from build123d import *

# Parameters (mm, degrees)
SKETCH1_W           = 20.32
SKETCH1_H           = 15.24
BOSS_EXTRUDE1_DEPTH = 5.4102
SKETCH2_W           = 10.414
SKETCH2_H           = 2.54
BOSS_EXTRUDE2_DEPTH = 8.382
SKETCH3_R           = 0.5715
CUT_EXTRUDE1_DEPTH  = 5.4102


with BuildPart() as part:
    # Sketch1 → Boss-Extrude1 (new body)
    with BuildSketch(Plane(origin=(0, 0, 0), x_dir=(1, 0, 0), z_dir=(0, 1, 0))):
        with Locations((10.16, 7.62)):
            Rectangle(SKETCH1_W, SKETCH1_H)
    extrude(amount=BOSS_EXTRUDE1_DEPTH)

    # Sketch2 → Boss-Extrude2 (add)
    with BuildSketch(Plane(origin=(0, 5.4102, 0), x_dir=(1, 0, 0), z_dir=(0, 1, 0))):
        with Locations((10.16, 12.7254)):
            Rectangle(SKETCH2_W, SKETCH2_H)
        with Locations((10.16, 2.5146)):
            Rectangle(SKETCH2_W, SKETCH2_H)
    extrude(amount=BOSS_EXTRUDE2_DEPTH)

    # Sketch3 → Cut-Extrude1 (cut)
    with BuildSketch(Plane.XZ):
        with Locations(Location((4.2545, -1.8161, 0), (0, 0, 270))):
            Circle(SKETCH3_R)
        with Locations(Location((16.0655, -1.8161, 0), (0, 0, 270))):
            Circle(SKETCH3_R)
        with Locations(Location((16.0655, -13.4239, 0), (0, 0, 270))):
            Circle(SKETCH3_R)
        with Locations(Location((4.2545, -13.4239, 0), (0, 0, 270))):
            Circle(SKETCH3_R)
    extrude(amount=-CUT_EXTRUDE1_DEPTH, mode=Mode.SUBTRACT)


solid = part.part
Here's how the part is built. I have some questions about the finished solid (model axes, mm). A direction names the side the tool comes from. Round coordinates to 2 decimals unless told otherwise and drop trailing zeros. Write each loop counter-clockwise with the first axis right and the second up, starting at its lowest first coordinate (ties: lowest second). Pieces come first, ordered by that corner, then holes.
1. Will these pins go through, and if not, where does the flat tip stop? pin 1 Ø4 at (x, y) = (9.5, 11.5) entering from -Z; pin 2 Ø0.8 at (y, z) = (9, -12.5) entering from -X; pin 3 Ø2.5 at (x, y) = (10.5, 8.5) entering from +Z.
2. Suppose I cut it at D-D (x = 4). List the corners of the cut face in (y, z) for me, and give its area (3 significant figures).
3. I need wall thicknesses on L1, parallel to Z at x = 5, y = 6.5; L2, parallel to Y at x = 6, z = -8.75. Which ranges of each line are inside material? Lowest first, please.
4. Suppose I cut it at B-B (x = 11.25). List the corners of the cut face in (y, z) for me, and give its area (3 significant figures).
5. For faces 4 (the flat face through (4.953, 10, -13)), 5 (the flat face through (15.367, 10, -13)), 6 (the flat face through (10, 10, -13.995)), 7 (the flat face through (10, 10, -1.245)), 8 (the flat face through (10, 10, -11.455)), which set-ups out of +Z, -Z, +X, -X, +Y, -Y let a thin tool reach every point of the face, with its end or its side?
6. If we mould it in two halves opening along Z, with no side actions, what happens to faces 1 (the flat face through (15.367, 10, -2)), 2 (the flat face through (10, 5.41, -8)), 3 (the flat face through (10, 3, 0))? For each: released by +Z, released by -Z, zero draft, split by the parting line, or undercut.
7. Suppose I cut it at A-A (y = 6). List the corners of the cut face in (x, z) for me, and give its area (3 significant figures).
8. Suppose I cut it at C-C (z = -12). List the corners of the cut face in (x, y) for me.
Answer sheet:
1. pin 1: stops at z = -14
1. pin 2: stops at x = 4.95
1. pin 3: stops at z = -1.24
2. outline: (0, -15.24) - (5.41, -15.24) - (5.41, -13.94) - (0, -13.94) - close; (0, -12.91) - (5.41, -12.91) - (5.41, -2.33) - (0, -2.33) - close; (0, -1.3) - (5.41, -1.3) - (5.41, 0) - (0, 0) - close
2. area: 71.4 mm2
3. L1: z = -14 to -11.46, -3.78 to -1.24
3. L2: y = 0 to 5.41
4. outline: (0, -15.24) - (5.41, -15.24) - (5.41, -14) - (13.79, -14) - (13.79, -11.46) - (5.41, -11.46) - (5.41, -3.78) - (13.79, -3.78) - (13.79, -1.24) - (5.41, -1.24) - (5.41, 0) - (0, 0) - close
4. area: 125 mm2
5. face 4: +Z, -Z, -X, +Y
5. face 5: +Z, -Z, +X, +Y
5. face 6: -Z, +X, -X, +Y
5. face 7: +Z, +X, -X, +Y
5. face 8: +X, -X, +Y
6. face 1: zero draft
6. face 2: undercut
6. face 3: released by +Z
7. outline: (4.95, -14) - (15.37, -14) - (15.37, -11.46) - (4.95, -11.46) - close; (4.95, -3.78) - (15.37, -3.78) - (15.37, -1.24) - (4.95, -1.24) - close
7. area: 52.9 mm2
8. outline: (0, 0) - (20.32, 0) - (20.32, 5.41) - (15.37, 5.41) - (15.37, 13.79) - (4.95, 13.79) - (4.95, 5.41) - (0, 5.41) - close
